Geometry check sheet. Reference: the model listing, model coordinates, mm. Face numbers are marked on the shaded views. A direction names the side the tool comes from. Round coordinates to 2 decimals unless told otherwise and drop trailing zeros. Write each loop counter-clockwise with the first axis right and the second up, starting at its lowest first coordinate (ties: lowest second). Pieces come first, ordered by that corner, then holes. Notation, with made-up numbers: (-18.5, 47) -> (-9.5, 47) arc R31 ccw to (-9.5, 77) -> close; hole circle Ø9 at (19.5, 50). An arc over 180 degrees is marked (long way). Use a Markdown table: item, result.
```python
from build123d import *

# Parameters (mm, degrees)
CROQUIS1_W                          = 15.5
CROQUIS1_H                          = 23.6
CROQUIS1_R                          = 2.1
SALIENTE_EXTRUIR1_DEPTH             = 5
SALIENTE_EXTRUIR2_REACH             = 40.26
SALIENTE_EXTRUIR2_DIRECTION_2_REACH = 40.26
REDONDEO1_R                         = 2
REDONDEO2_R                         = 10
CHAFL_N1_SIZE                       = 1.5
CHAFL_N2_SIZE                       = 1.5


with BuildPart() as part:
    # Croquis1 → Saliente-Extruir1 (new body)
    with BuildSketch(Plane.XY):
        with Locations((28.3, 0)):
            Rectangle(CROQUIS1_W, CROQUIS1_H)
        with Locations((24.250000128, -5)):
            Circle(CROQUIS1_R, mode=Mode.SUBTRACT)
        with Locations((24.250000128, 5)):
            Circle(CROQUIS1_R, mode=Mode.SUBTRACT)
    extrude(amount=SALIENTE_EXTRUIR1_DEPTH)

    # Saliente-Extruir2: up to this face of the body (flat: up to its plane)
    saliente_extruir2_end = Plane(part.part.faces().sort_by_distance((28.3, -11.8, 2.5))[0])
    # Croquis2 → Saliente-Extruir2 (add, up to the picked face)
    with BuildSketch(Plane(origin=(0, 0, 0), x_dir=(1, 0, 0), z_dir=(0, 1, 0)), mode=Mode.PRIVATE) as saliente_extruir2_sk1:
        with BuildLine():
            ThreePointArc((39.254957851, 0), (55.312581622, -1.388967795), (58.268482288, 14.455247679))
            Line((58.268482288, 14.455247679), (58.268482288, 21.749894336))
            ThreePointArc((58.268482288, 21.749894336), (61.427658114, -2.326136764), (37.292908876, -5))
            Line((37.292908876, -5), (36.05, -5))
            Line((36.05, -5), (36.05, 0))
            Line((36.05, 0), (39.254957851, 0))
        make_face()
    saliente_extruir2_tool1 = split(extrude(saliente_extruir2_sk1.sketch, amount=-SALIENTE_EXTRUIR2_REACH, mode=Mode.PRIVATE), bisect_by=saliente_extruir2_end, keep=Keep.BOTH, mode=Mode.PRIVATE)
    add(saliente_extruir2_tool1.solids().sort_by(Axis((55.567672, 0, 1.724497), (0, -1, 0)))[0])

    # Saliente-Extruir2 direction 2: up to this face of the body (flat: up to its plane)
    saliente_extruir2_direction_2_end = Plane(part.part.faces().sort_by_distance((28.3, 11.8, 2.5))[0])
    # Croquis2 → Saliente-Extruir2 direction 2 (add, up to the picked face)
    with BuildSketch(Plane(origin=(0, 0, 0), x_dir=(1, 0, 0), z_dir=(0, 1, 0)), mode=Mode.PRIVATE) as saliente_extruir2_direction_2_sk1:
        with BuildLine():
            ThreePointArc((39.254957851, 0), (55.312581622, -1.388967795), (58.268482288, 14.455247679))
            Line((58.268482288, 14.455247679), (58.268482288, 21.749894336))
            ThreePointArc((58.268482288, 21.749894336), (61.427658114, -2.326136764), (37.292908876, -5))
            Line((37.292908876, -5), (36.05, -5))
            Line((36.05, -5), (36.05, 0))
            Line((36.05, 0), (39.254957851, 0))
        make_face()
    saliente_extruir2_direction_2_tool1 = split(extrude(saliente_extruir2_direction_2_sk1.sketch, amount=SALIENTE_EXTRUIR2_DIRECTION_2_REACH, mode=Mode.PRIVATE), bisect_by=saliente_extruir2_direction_2_end, keep=Keep.BOTH, mode=Mode.PRIVATE)
    add(saliente_extruir2_direction_2_tool1.solids().sort_by(Axis((55.567672, 0, 1.724497), (0, 1, 0)))[0])

    # Redondeo1
    redondeo1_edges = [part.edges().sort_by_distance(p)[0] for p in [
        (58.268482288, 0, -21.749894336),
        (39.254957851, 0, 0),
    ]]
    fillet(redondeo1_edges, radius=REDONDEO1_R)

    # Redondeo2
    redondeo2_edges = [part.edges().sort_by_distance(p)[0] for p in [
        (37.292908876, 0, 5),
    ]]
    fillet(redondeo2_edges, radius=REDONDEO2_R)

    # Chaflán1
    chafl_n1_edges = [part.edges().sort_by_distance(p)[0] for p in [
        (58.268482288, 11.8, -15.660048739),
        (55.615767212, -11.8, 1.150684381),
        (58.268482288, -11.8, -15.660048739),
        (55.615767212, 11.8, 1.150684381),
        (29.486018705, 11.8, 0),
        (60.537424453, 11.8, 3.37157131),
        (59.659492117, 11.8, -18.769877613),
        (39.162329274, 11.8, 0.142052757),
        (60.537424453, -11.8, 3.37157131),
        (59.659492117, -11.8, -18.769877613),
        (39.162329274, -11.8, 0.142052757),
        (27.363871837, 11.8, 5),
        (36.843099013, 11.8, 5.361749074),
        (36.843099013, -11.8, 5.361749074),
        (29.486018705, -11.8, 0),
        (27.363871837, -11.8, 5),
        (20.55, 11.8, 2.5),
        (20.55, -11.8, 2.5),
    ]]
    chamfer(chafl_n1_edges, length=CHAFL_N1_SIZE)

    # Chaflán2
    chafl_n2_edges = [part.edges().sort_by_distance(p)[0] for p in [
        (22.150000128, -5, 5),
        (22.150000128, 5, 5),
    ]]
    chamfer(chafl_n2_edges, length=CHAFL_N2_SIZE)


solid = part.part
```
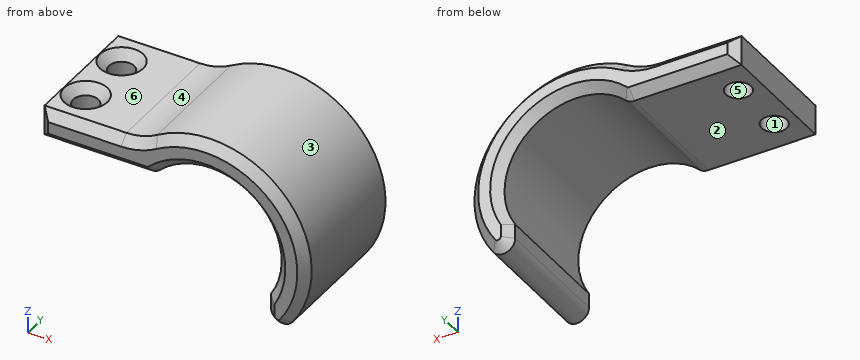
(1) Section check C-C on y = -9.25. Record the cut outline in (x, z) (3 decimals).
A:
| item | result |
|---|---|
| outline | (20.55, 0) -> (38.422, 0) arc R2 ccw to (39.797, 0.548) arc R12 cw to (58.268, -14.455) -> (58.268, -16.865) arc R2 ccw to (61.898, -18.025) arc R17 ccw to (39.316, 6.421) arc R10 cw to (34.178, 5) -> (20.55, 5) -> close |
(2) Section check B-B on y = 5. Record the cut outline in (x, z) (3 decimals).
A:
| item | result |
|---|---|
| outline | (20.55, 0) -> (22.15, 0) -> (22.15, 3.5) -> (20.65, 5) -> (20.55, 5) -> close; (26.35, 0) -> (38.422, 0) arc R2 ccw to (39.797, 0.548) arc R12 cw to (58.268, -14.455) -> (58.268, -16.865) arc R2 ccw to (61.898, -18.025) arc R17 ccw to (39.316, 6.421) arc R10 cw to (34.178, 5) -> (27.85, 5) -> (26.35, 3.5) -> close |
(3) Section check D-D on x = 33. Record the cut outline in (y, z).
A:
| item | result |
|---|---|
| outline | (-11.8, 1.5) -> (-10.3, 0) -> (10.3, 0) -> (11.8, 1.5) -> (11.8, 3.5) -> (10.3, 5) -> (-10.3, 5) -> (-11.8, 3.5) -> close |
(4) Release check for a two-part mould opening along X. For the marked faces 3, 4, 5 and 6 record: +X half, -X half, draft (parallel to the pull), parting line (faces both ways), or undercut.
A:
| item | result |
|---|---|
| face 3 | parting line |
| face 4 | -X half |
| face 5 | undercut |
| face 6 | draft |
(5) Thickness scan on line 1 (Y direction, x = 24.25, z = 2.6); line 2 (Y direction, x = 24.25, z = 1.1); line 3 (Z direction, x = 48, y = 1.5). Record the ranges inside material, lowest first.
A:
| item | result |
|---|---|
| line 1 | y = -11.8 to -7.1, -2.9 to 2.9, 7.1 to 11.8 |
| line 2 | y = -11.4 to -7.1, -2.9 to 2.9, 7.1 to 11.4 |
| line 3 | z = 3.84 to 8.84 |
(6) Access from +Z, -Z, +X, -X, +Y, -Y to the whole of each face (thin tool, end or side, straight path). Record for the marked faces 1 and 2.
A:
| item | result |
|---|---|
| face 1 | +Z, -Z |
| face 2 | -Z, -X, +Y, -Y |
(7) Gauge pin test, flat ends, axial feed: pin 1 Ø5 at (x, y) = (24.25, -5) entering from -Z; pin 2 Ø4 at (x, y) = (40, 7.5) entering from +Z; pin 3 Ø4 at (x, y) = (38, 4) entering from +Z. Record the tip position at first contact, or that the pin passes through.
A:
| item | result |
|---|---|
| pin 1 | stops at z = 0 |
| pin 2 | stops at z = 7.72 |
| pin 3 | stops at z = 6.81 |
(8) Section check A-A on x = 24.25. Record the cut outline in (y, z).
A:
| item | result |
|---|---|
| outline | (-11.8, 1.5) -> (-10.3, 0) -> (-7.1, 0) -> (-7.1, 3.5) -> (-8.6, 5) -> (-10.3, 5) -> (-11.8, 3.5) -> close; (-2.9, 0) -> (2.9, 0) -> (2.9, 3.5) -> (1.4, 5) -> (-1.4, 5) -> (-2.9, 3.5) -> close; (7.1, 0) -> (10.3, 0) -> (11.8, 1.5) -> (11.8, 3.5) -> (10.3, 5) -> (8.6, 5) -> (7.1, 3.5) -> close |
